For this review, take the finished solid that the model builds, in its own axes (mm). Face numbers are marked on the shaded views. Coordinates: 2 decimals unless noted, no trailing zeros. Order: outer loops, then holes, each group sorted by start corner. A loop starts at its lowest first (then second) coordinate and runs counter-clockwise, first axis right, second up. Notation, with made-up numbers: (-34, 83) -> (-30, 83) arc R16 ccw to (-30, 97) -> close; hole circle Ø9 at (0.5, -22). An arc over 180 degrees is marked (long way). Return JSON: item names as keys, results as strings. Group by question number.
Item 1: Take a section at D-D (x = 2). Write out the cut boundary in (y, z), then the cut area to 3 significant figures.
Item 2: For line 1 along Y through (x, z) = (0.05, 2.45); line 2 along Y through (x, z) = (0, 0.8); line 3 along X through (y, z) = (6.5, -0.1), list the stretches that pass through material, from the lowest coordinate up.
Item 3: Take a section at B-B (y = 6.25). Write out the cut boundary in (x, z), then the cut area to 3 significant figures.
Item 4: Draft analysis for pull direction X (two halves, no side actions). For the marked faces 1, 2 and 3, state which applies: +X half, -X half, draft (parallel to the pull), parting line (faces both ways), or undercut.
Item 5: Insertion check: pin 1 (1 mm diameter, centred on x = 2, z = -0.5, fed in from +Y); pin 2 (3 mm diameter, centred on x = 0, y = 6.5, fed in from -Z). Each pin has a flat end and moves straight along its axis. Give the tip position at first contact, or say it passes through.
Item 6: Take a section at A-A (z = 0). Write out the cut boundary in (x, y), then the cut area to 3 significant figures.
Item 7: Take a section at C-C (x = -2.2). Write out the cut boundary in (y, z), then the cut area to 3 significant figures.
```python
from build123d import *

# Parameters (mm, degrees)
SKETCH_1_R          = 2.75
EXTRUDE_1_DEPTH     = 3
CUT_EXTRUDE_1_DEPTH = 1.5
SKETCH_2_R          = 1.5
EXTRUDE_2_DEPTH     = 10
CHAMFER_1_SIZE      = 0.3


with BuildPart() as part:
    # 草图1 → 凸台-拉伸1 (new body)
    with BuildSketch(Plane(origin=(0, 0, 0), x_dir=(1, 0, 0), z_dir=(0, 1, 0))):
        with Locations(Location((0, 0, 0), (0, 0, 270))):
            Circle(SKETCH_1_R)
    extrude(amount=EXTRUDE_1_DEPTH)

    # 草图3 → 切除-拉伸1 (cut)
    with BuildSketch(Plane.XZ):
        Polygon((0, 1.25), (-1.082531755, 0.625), (-1.082531755, -0.625), (0, -1.25), (1.082531755, -0.625), (1.082531755, 0.625), align=None)
    extrude(amount=-CUT_EXTRUDE_1_DEPTH, mode=Mode.SUBTRACT)

    # 草图2 → 凸台-拉伸2 (add)
    with BuildSketch(Plane(origin=(0, 3, 0), x_dir=(1, 0, 0), z_dir=(0, 1, 0))):
        with Locations(Location((0, 0, 0), (0, 0, 270))):
            Circle(SKETCH_2_R)
    extrude(amount=EXTRUDE_2_DEPTH)

    # 倒角1
    chamfer_1_edges = [part.edges().sort_by_distance(p)[0] for p in [
        (0, 13, -1.5),
    ]]
    chamfer(chamfer_1_edges, length=CHAMFER_1_SIZE)


solid = part.part
```
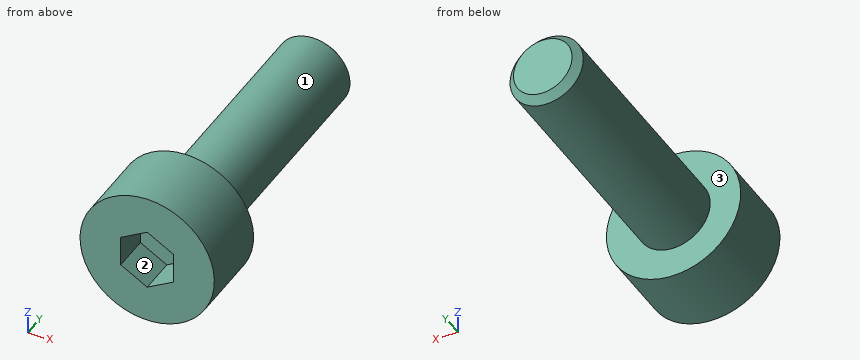
Findings below:
{
 "1": {"outline": "(0, -1.89) -> (3, -1.89) -> (3, 1.89) -> (0, 1.89) -> close", "area": "11.3 mm2"},
 "2": {"line 1": "y = 0 to 3", "line 2": "y = 1.5 to 13", "line 3": "x = -1.5 to 1.5"},
 "3": {"outline": "circle Ø3 at (0, 0)", "area": "7.07 mm2"},
 "4": {"face 1": "parting line", "face 2": "undercut", "face 3": "draft"},
 "5": {"pin 1": "stops at y = 3", "pin 2": "stops at z = -1.5"},
 "6": {"outline": "(-2.75, 0) -> (-1.08, 0) -> (-1.08, 1.5) -> (1.08, 1.5) -> (1.08, 0) -> (2.75, 0) -> (2.75, 3) -> (1.5, 3) -> (1.5, 12.7) -> (1.2, 13) -> (-1.2, 13) -> (-1.5, 12.7) -> (-1.5, 3) -> (-2.75, 3) -> close", "area": "43.2 mm2"},
 "7": {"outline": "(0, -1.65) -> (3, -1.65) -> (3, 1.65) -> (0, 1.65) -> close", "area": "9.90 mm2"}
}
